Verification items for the finished model (mm, model axes). Round coordinates to 2 decimals unless told otherwise and drop trailing zeros. Write each loop counter-clockwise with the first axis right and the second up, starting at its lowest first coordinate (ties: lowest second). Pieces come first, ordered by that corner, then holes. Notation, with made-up numbers: (33, 59.5) -> (52, 59.5) arc R18 ccw to (52, 79.5) -> close; hole circle Ø10 at (-5.75, -21). An arc over 180 degrees is marked (long way). Use CSV: the item, a comma, the result in double quotes.
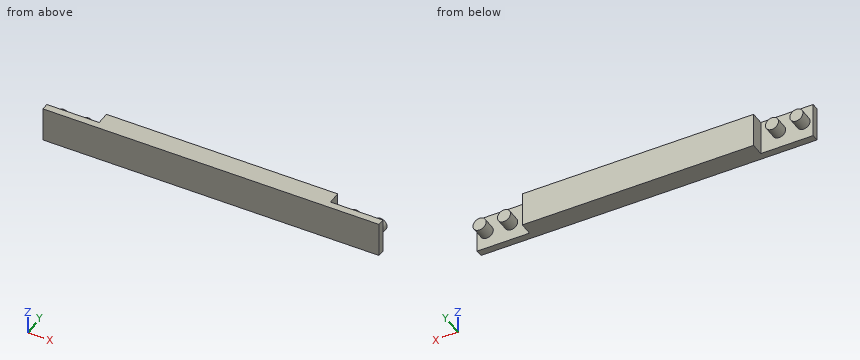
```python
from build123d import *

# Parameters (mm, degrees)
SKETCH_1_W      = 26.5
SKETCH_1_H      = 4
SKETCH_1_W_2    = 6
EXTRUDE_1_DEPTH = 0.8
EXTRUDE_START   = 0.8
SKETCH_1_3_W    = 26.5
SKETCH_1_3_H    = 4
EXTRUDE_2_DEPTH = 1.5
SKETCH_2_R      = 0.75
EXTRUDE_3_DEPTH = 1.5


with BuildPart() as part:
    # Эскиз1 → Бобышка-Вытянуть1 (new body)
    with BuildSketch(Plane(origin=(0, 0, 0), x_dir=(1, 0, 0), z_dir=(0, 1, 0))):
        Rectangle(SKETCH_1_W, SKETCH_1_H)
        with Locations((-16.25, 0)):
            Rectangle(SKETCH_1_W_2, SKETCH_1_H)
        with Locations((16.25, 0)):
            Rectangle(SKETCH_1_W_2, SKETCH_1_H)
    extrude(amount=EXTRUDE_1_DEPTH)

    # Эскиз1<3> → Бобышка-Вытянуть2 (add)
    with BuildSketch(Plane(origin=(0, 0, 0), x_dir=(1, 0, 0), z_dir=(0, 1, 0)).offset(EXTRUDE_START)):
        Rectangle(SKETCH_1_3_W, SKETCH_1_3_H)
    extrude(amount=EXTRUDE_2_DEPTH)

    # Эскиз2 → Бобышка-Вытянуть3 (add)
    with BuildSketch(Plane(origin=(0, 0.8, 0), x_dir=(1, 0, 0), z_dir=(0, 1, 0))):
        with Locations(Location((-15.35, 0, 0), (0, 0, 270))):
            Circle(SKETCH_2_R)
        with Locations(Location((-18.15, 0, 0), (0, 0, 270))):
            Circle(SKETCH_2_R)
        with Locations(Location((18.15, 0, 0), (0, 0, 90))):
            Circle(SKETCH_2_R)
        with Locations(Location((15.35, 0, 0), (0, 0, 90))):
            Circle(SKETCH_2_R)
    extrude(amount=EXTRUDE_3_DEPTH)


solid = part.part
```
Q1. Section check B-B (z = 0). Record the cut outline in (x, y).
Filled in:
outline,"(-19.25, 0) -> (19.25, 0) -> (19.25, 0.8) -> (18.9, 0.8) -> (18.9, 2.3) -> (17.4, 2.3) -> (17.4, 0.8) -> (16.1, 0.8) -> (16.1, 2.3) -> (14.6, 2.3) -> (14.6, 0.8) -> (13.25, 0.8) -> (13.25, 2.3) -> (-13.25, 2.3) -> (-13.25, 0.8) -> (-14.6, 0.8) -> (-14.6, 2.3) -> (-16.1, 2.3) -> (-16.1, 0.8) -> (-17.4, 0.8) -> (-17.4, 2.3) -> (-18.9, 2.3) -> (-18.9, 0.8) -> (-19.25, 0.8) -> close"
Q2. Go/stop test with flat-tipped pins: P1, Ø0.7, axis at y = 1.5, z = 0.5, coming from the +X side; P2, Ø1, axis at x = -14, y = 1.5, coming from the -Z side. Record where each tip stops, or that it passes through.
Filled in:
P1,"x = 18.88"
P2,"through"
Q3. Section check D-D (x = 15). Record the cut outline in (y, z).
Filled in:
outline,"(0, -2) -> (0.8, -2) -> (0.8, -0.66) -> (2.3, -0.66) -> (2.3, 0.66) -> (0.8, 0.66) -> (0.8, 2) -> (0, 2) -> close"
Q4. Material ranges on L1, parallel to X at y = 1.9, z = 0; L2, parallel to X at y = 1.4, z = 0.3; L3, parallel to X at y = 1.75, z = -1.3, recorded low to high.
Filled in:
L1,"-18.9 to -17.4, -16.1 to -14.6, -13.25 to 13.25, 14.6 to 16.1, 17.4 to 18.9"
L2,"-18.84 to -17.46, -16.04 to -14.66, -13.25 to 13.25, 14.66 to 16.04, 17.46 to 18.84"
L3,"-13.25 to 13.25"
Q5. Section check A-A (y = 1.45). Record the cut outline in (x, z).
Filled in:
outline,"circle Ø1.5 at (-18.15, 0); circle Ø1.5 at (-15.35, 0); (-13.25, -2) -> (13.25, -2) -> (13.25, 2) -> (-13.25, 2) -> close; circle Ø1.5 at (15.35, 0); circle Ø1.5 at (18.15, 0)"
Q6. Section check C-C (x = -18.15). Record the cut outline in (y, z).
Filled in:
outline,"(0, -2) -> (0.8, -2) -> (0.8, -0.75) -> (2.3, -0.75) -> (2.3, 0.75) -> (0.8, 0.75) -> (0.8, 2) -> (0, 2) -> close"
